For this review, take the finished solid that the model builds, in its own axes (mm). Face numbers are marked on the shaded views. A direction names the side the tool comes from. Round coordinates to 2 decimals unless told otherwise and drop trailing zeros. Order: outer loops, then holes, each group sorted by start corner. A loop starts at its lowest first (then second) coordinate and runs counter-clockwise, first axis right, second up. Notation, with made-up numbers: M 77.25,50.25 L 123.25,50.25 A19 ccw 123.25,63.25 Z; hole C 73.5,2.25 d5. An arc over 180 degrees is marked long. Answer in a Markdown table with one row per item. Add a question column.
```python
from build123d import *

# Parameters (mm, degrees)
F1_DEPTH = 101.6
F2_R     = 3.175
F3_R     = 2.413


with BuildPart() as f1:
    # F0 (on Right) → F1 (new body)
    with BuildSketch(Plane.YZ):
        Polygon((79.375, 0), (0, 0), (0, -79.375), (4.7625, -79.375), (4.7625, -4.7625), (79.375, -4.7625), align=None)
    extrude(amount=F1_DEPTH)

    # F2
    f2_edges = [f1.edges().sort_by_distance(p)[0] for p in [
        (50.8, 0, 0),
    ]]
    fillet(f2_edges, radius=F2_R)

    # F3
    f3_edges = [f1.edges().sort_by_distance(p)[0] for p in [
        (50.8, 4.7625, -4.7625),
    ]]
    fillet(f3_edges, radius=F3_R)


solid = f1.part
```
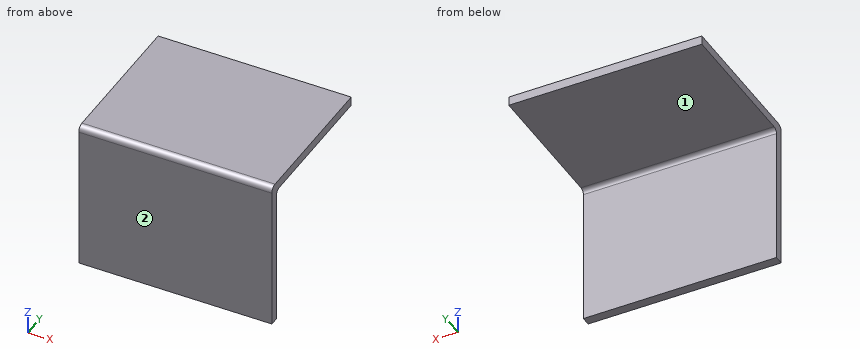
1. Consider section C-C on z = -53. Write out the cut boundary in (x, y), plus the area to 3 significant figures.
2. Clearance check with flat-ended pins moving along their axes: pin 1 Ø12 at (x, y) = (15, 19.5) entering from -Z; pin 2 Ø21.5 at (x, z) = (72, -42) entering from +Y. State where each tip first meets the part, or that it passes through.
3. To check wall thickness, follow probe 1 along Z at (x, y) = (67.5, 18.5); probe 2 along Y at (x, z) = (44, -61.5); probe 3 along Z at (x, y) = (56.5, 5.5). State the ranges of each line that lie inside material, in increasing order. Write a range as [from, to].
4. Consider section B-B on y = 22. Write out the cut boundary in (x, z).
5. For the marked faces 1 and 2, list the 3-axis set-ups (+Z, -Z, +X, -X, +Y, -Y) from which the entire face can be reached by the end or side of a thin tool; tool diameter is ignored.
Solved:
| question | item | result |
|---|---|---|
| 1 | outline | M 0,0 L 101.6,0 L 101.6,4.76 L 0,4.76 Z |
| 1 | area | 484 mm^2 |
| 2 | pin 1 | stops at z = -4.76 |
| 2 | pin 2 | stops at y = 4.76 |
| 3 | probe 1 | z = [-4.76, 0] |
| 3 | probe 2 | y = [0, 4.76] |
| 3 | probe 3 | z = [-5.44, 0] |
| 4 | outline | M 0,-4.76 L 101.6,-4.76 L 101.6,0 L 0,0 Z |
| 5 | face 1 | -Z, +X, -X, +Y |
| 5 | face 2 | +Z, -Z, +X, -X, -Y |
